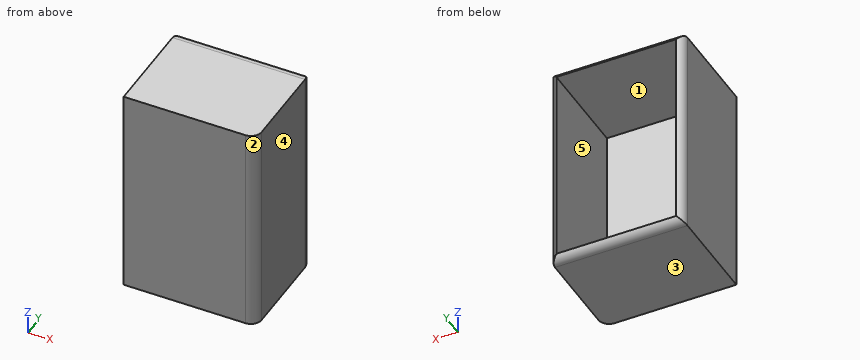
```python
from build123d import *

# Parameters (mm, degrees)
F0_W        = 63.2100254297
F0_H        = 50.6872721016
F1_DEPTH    = 101.6
F2_T        = -3.048
F3_T1_DEPTH = 127
F3_T3_DEPTH = 88.6100254297


# Not quite as in the source:
# - a fillet or chamfer that OpenCascade refuses, or shapes differently, is made with other operations: its cross-section is extruded or revolved along the edge and cut away or added


with BuildPart() as f1:
    # F0 (on Top) → F1 (new body)
    with BuildSketch(Plane.XY):
        with Locations((31.6050127149, -25.3436360508)):
            Rectangle(F0_W, F0_H)
    extrude(amount=F1_DEPTH)

    # F2
    f2_openings = [f1.faces().sort_by_distance(p)[0] for p in [
        (31.605013, 0, 50.8),
    ]]
    offset(amount=F2_T, openings=f2_openings)

    # F3: fillet of radius 5.08 on 5 edges, made by hand

    # F3_s2 → F3_t1 (cut)
    with BuildSketch(Plane.XY.offset(-12.7)):
        with BuildLine():
            ThreePointArc((0, -5.08), (1.4878975516, -1.4878975516), (5.08, 0))
            Line((5.08, 0), (0, 0))
            Line((0, 0), (0, -5.08))
        make_face()
        with BuildLine():
            ThreePointArc((63.2100254297, -5.08), (61.7221278782, -1.4878975516), (58.1300254297, 0))
            Line((58.1300254297, 0), (63.2100254297, 0))
            Line((63.2100254297, 0), (63.2100254297, -5.08))
        make_face()
        with BuildLine():
            ThreePointArc((58.1300254297, -50.6872721016), (61.7221278782, -49.1993745501), (63.2100254297, -45.6072721016))
            Line((63.2100254297, -45.6072721016), (63.2100254297, -50.6872721016))
            Line((63.2100254297, -50.6872721016), (58.1300254297, -50.6872721016))
        make_face()
    extrude(amount=F3_T1_DEPTH, mode=Mode.SUBTRACT)

    # F3_s4 → F3_t3 (cut)
    with BuildSketch(Plane.YZ.offset(-12.7)):
        with BuildLine():
            ThreePointArc((-5.08, 101.6), (-1.4878975516, 100.1121024484), (0, 96.52))
            Line((0, 96.52), (0, 101.6))
            Line((0, 101.6), (-5.08, 101.6))
        make_face()
        with BuildLine():
            ThreePointArc((-5.08, 0), (-1.4878975516, 1.4878975516), (0, 5.08))
            Line((0, 5.08), (0, 0))
            Line((0, 0), (-5.08, 0))
        make_face()
    extrude(amount=F3_T3_DEPTH, mode=Mode.SUBTRACT)


solid = f1.part
```
Can you work these out from the model? Positions are in its coordinate system, mm. Face numbers are marked on the shaded views. A direction names the side the tool comes from. Round coordinates to 2 decimals unless told otherwise and drop trailing zeros. Loops run counter-clockwise (first coordinate to the right, second up) from the corner with the lowest first, then second, coordinate; pieces in that order, holes last. Notation, with made-up numbers: (-6, 19.25) -> (26, 19.25) arc R23 ccw to (26, 49.25) -> close; hole circle Ø1 at (17.25, 8.25). An arc over 180 degrees is marked (long way). One line per item, written item: value. Start each with the question number.
1. If I drill on probe 1 along X at (y, z) = (-35, 42); probe 2 along Z at (x, y) = (49.5, -32); probe 3 along Y at (x, z) = (19.5, 12), over which ranges is the centre line in solid material (lowest first)?
2. If we section it at A-A, the plane y = -39: Write out the boundary of the cut face in (x, z), then the cut area to 3 significant figures.
3. If we section it at B-B, the plane z = 31.5: Write out the boundary of the cut face in (x, y).
4. If we mould it in two halves opening along Z, with no side actions, what happens to the marked faces 1, 2 and 3? For each: pulls with the +Z half, pulls with the -Z half, needs draft (parallel to the pull), parting line crosses it, or undercut.
5. For pin 1 (10 mm diameter, centred on x = 30.5, z = 86.5, fed in from +Y); pin 2 (3 mm diameter, centred on x = 29.5, y = -45, fed in from -Z), each with a flat end and sliding along its axis, tell me the tip position at first contact or that it passes through.
6. If we section it at C-C, the plane x = 39: Write out the boundary of the cut face in (y, z).
7. For the marked faces 4 and 5, which set-ups out of +Z, -Z, +X, -X, +Y, -Y let a thin tool reach every point of the face, with its end or its side?
Calculated:
1. probe 1: x = 0 to 3.05, 60.16 to 63.21
1. probe 2: z = 0 to 3.05, 98.55 to 101.6
1. probe 3: y = -50.69 to -47.64
2. outline: (0, 0) -> (63.21, 0) -> (63.21, 101.6) -> (0, 101.6) -> close; hole (3.05, 3.05) -> (60.16, 3.05) -> (60.16, 98.55) -> (3.05, 98.55) -> close
2. area: 968 mm²
3. outline: (0, -50.69) -> (58.13, -50.69) arc R5.08 ccw to (63.21, -45.61) -> (63.21, -5.08) arc R5.08 ccw to (60.16, -0.42) -> (60.16, -47.64) -> (3.05, -47.64) -> (3.05, -0.42) arc R5.08 ccw to (0, -5.08) -> close
4. face 1: undercut
4. face 2: needs draft
4. face 3: pulls with the -Z half
5. pin 1: stops at y = -47.64
5. pin 2: stops at z = 0
6. outline: (-50.69, 0) -> (-5.08, 0) arc R5.08 ccw to (-0.42, 3.05) -> (-47.64, 3.05) -> (-47.64, 98.55) -> (-0.42, 98.55) arc R5.08 ccw to (-5.08, 101.6) -> (-50.69, 101.6) -> close
7. face 4: +Z, -Z, +X, +Y, -Y
7. face 5: +Y
